```python
from build123d import *

# Parameters (mm, degrees)
SKETCH1_W                = 14.5
SKETCH1_H                = 18
BOSS_EXTRUDE1_DEPTH      = 1.5
BOSS_EXTRUDE2_DEPTH      = 4
BOSS_EXTRUDE2_DEPTH_BACK = 7
SKETCH2_R                = 3
SKETCH3_R                = 1.5
CUT_EXTRUDE1_DEPTH       = 1
SKETCH4_W                = 2
SKETCH4_H                = 6
BOSS_EXTRUDE3_DEPTH      = 6.5
SKETCH5_W                = 7.62
SKETCH5_H                = 2.54
BOSS_EXTRUDE4_DEPTH      = 3
SKETCH7_R                = 1.25
CUT_EXTRUDE2_DEPTH       = 17.242305871


with BuildPart() as part:
    # Sketch1 → Boss-Extrude1 (new body)
    with BuildSketch(Plane(origin=(0, 0, 0), x_dir=(1, 0, 0), z_dir=(0, 1, 0))):
        Rectangle(SKETCH1_W, SKETCH1_H)
    extrude(amount=BOSS_EXTRUDE1_DEPTH)



with BuildPart() as body_2:
    # Sketch2 → Boss-Extrude2 (new, two sides: drawn at the far end of the back side and taken through both)
    with BuildSketch(Plane.XY.offset(9).offset(-BOSS_EXTRUDE2_DEPTH_BACK)):
        with Locations((0, 5)):
            Circle(SKETCH2_R)
    extrude(amount=BOSS_EXTRUDE2_DEPTH + BOSS_EXTRUDE2_DEPTH_BACK)

    # Sketch3 → Cut-Extrude1 (cut)
    with BuildSketch(Plane.XY.offset(13)):
        with Locations((0, 5)):
            Circle(SKETCH3_R)
    extrude(amount=-CUT_EXTRUDE1_DEPTH, mode=Mode.SUBTRACT)


with BuildPart() as part_1:
    add(part.part)

    add(body_2.part)  # Boss-Extrude3 merges body 2
    # Sketch4 → Boss-Extrude3 (add)
    with BuildSketch(Plane(origin=(0, 1.5, 0), x_dir=(1, 0, 0), z_dir=(0, 1, 0))):
        with Locations((0, -2)):
            Rectangle(SKETCH4_W, SKETCH4_H)
    extrude(amount=BOSS_EXTRUDE3_DEPTH)

    # Sketch5 → Boss-Extrude4 (add)
    with BuildSketch(Plane(origin=(0, 1.5, 0), x_dir=(1, 0, 0), z_dir=(0, 1, 0))):
        with Locations((0, 7.23)):
            Rectangle(SKETCH5_W, SKETCH5_H)
    extrude(amount=BOSS_EXTRUDE4_DEPTH)

    # Sketch7 → Cut-Extrude2 (cut, through all)
    with BuildSketch(Plane(origin=(0, 1.5, 0), x_dir=(1, 0, 0), z_dir=(0, 1, 0))):
        with Locations(Location((-5.5, -4.25, 0), (0, 0, 270))):
            Circle(SKETCH7_R)
        with Locations(Location((5.5, -4.25, 0), (0, 0, 90))):
            Circle(SKETCH7_R)
    extrude(amount=-CUT_EXTRUDE2_DEPTH, mode=Mode.SUBTRACT)


solid = part_1.part
```
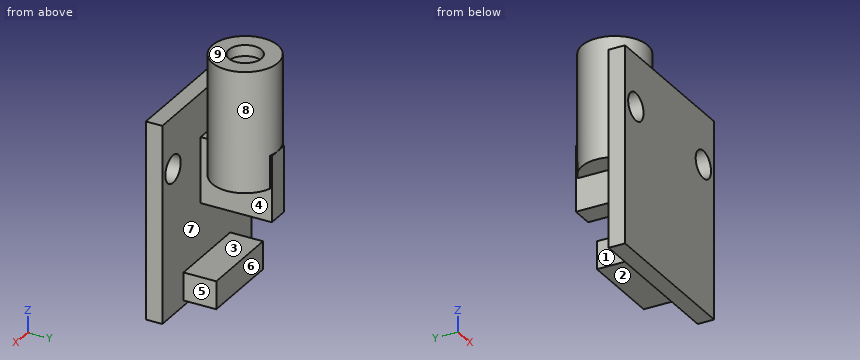
For this review, take the finished solid that the model builds, in its own axes (mm). Face numbers are marked on the shaded views. A direction names the side the tool comes from. Round coordinates to 2 decimals unless told otherwise and drop trailing zeros. Write each loop counter-clockwise with the first axis right and the second up, starting at its lowest first coordinate (ties: lowest second). Pieces come first, ordered by that corner, then holes. Notation, with made-up numbers: (-40, 34.25) -> (12, 34.25) arc R27 ccw to (12, 52.25) -> close; hole circle Ø8 at (12.5, -0.5). An arc over 180 degrees is marked (long way). Use one line per item in the form item = value.
1) To check wall thickness, follow L1, parallel to X at y = 1.1, z = 4.25; L2, parallel to Z at x = 0.25, y = 3; L3, parallel to Z at x = -2, y = 0.75. State the ranges of each line that lie inside material, in increasing order. Write a range as from..to.
Found:
L1 = -7.25..-6.75, -4.25..4.25, 6.75..7.25
L2 = -8.5..-5.96, -1..13
L3 = -9..9
2) Tool access review of the marked faces 1, 2, 3, 4 and 5: name each direction out of +Z, -Z, +X, -X, +Y, -Y from which nothing blocks a thin tool from reaching the whole face with its end or side.
Found:
face_1 = +Z, -Z, -X, +Y
face_2 = -Z, +X, -X, +Y
face_3 = +X, -X, +Y
face_4 = +X
face_5 = +Z, -Z, +X, +Y
3) Clearance check with flat-ended pins moving along their axes: pin 1 (3 mm diameter, centred on x = -5.5, z = 4.25, fed in from +Y); pin 2 (0.6 mm diameter, centred on x = 0, y = 5, fed in from -Z); pin 3 (1.6 mm diameter, centred on x = 2, y = 3.5, fed in from -Z). State where each tip first meets the part, or that it passes through.
Found:
pin_1 = 1.5
pin_2 = -1
pin_3 = -8.5
4) Take a section at D-D, the plane y = 5. Write out the cut boundary in (x, z).
Found:
outline = (-3, 2) -> (-1, 2) -> (-1, -1) -> (1, -1) -> (1, 2) -> (3, 2) -> (3, 13) -> (1.5, 13) -> (1.5, 12) -> (-1.5, 12) -> (-1.5, 13) -> (-3, 13) -> close
5) Take a section at B-B, the plane y = 1.75. Write out the cut boundary in (x, z), and give its area (3 significant figures).
Found:
outline = (-3.81, -8.5) -> (3.81, -8.5) -> (3.81, -5.96) -> (-3.81, -5.96) -> close; (-1, -1) -> (1, -1) -> (1, 5) -> (-1, 5) -> close
area = 31.4 mm2
6) Mouldability with a two-part tool opening along Y and no side actions: class the marked faces 6, 7, 8 and 9 as +Y half, -Y half, draft (parallel to the pull), parting line (faces both ways), or undercut.
Found:
face_6 = +Y half
face_7 = undercut
face_8 = undercut
face_9 = draft
7) Take a section at A-A, the plane x = 5.5. Write out the cut boundary in (y, z).
Found:
outline = (0, -9) -> (1.5, -9) -> (1.5, 3) -> (0, 3) -> close; (0, 5.5) -> (1.5, 5.5) -> (1.5, 9) -> (0, 9) -> close
8) Take a section at C-C, the plane z = -0.5. Write out the cut boundary in (x, y), and give its area (4 significant figures).
Found:
outline = (-7.25, 0) -> (7.25, 0) -> (7.25, 1.5) -> (1, 1.5) -> (1, 8) -> (-1, 8) -> (-1, 1.5) -> (-7.25, 1.5) -> close
area = 34.75 mm2
